```python
from build123d import *

# Parameters (mm, degrees)
SKETCH1_W = 9.525
SKETCH1_H = 3.175


with BuildPart() as part:
    # Sketch1 → Revolve2 (revolve)
    with BuildSketch(Plane.XY, mode=Mode.PRIVATE) as revolve2_sk:
        Polygon((0, 9.525), (0, 0), (31.75, 0), (31.75, 7.62), (31.75, 9.525), align=None)
        Polygon((31.75, 7.62), (31.75, 0), (38.1, 0), (38.1, 6.35), (38.1, 7.62), align=None)
        Polygon((38.1, 6.35), (38.1, 0), (47.625, 0), (47.625, 5.715), (47.625, 6.35), align=None)
        Polygon((47.625, 5.715), (47.625, 0), (57.15, 0), (57.15, 4.445), (57.15, 5.715), align=None)
        Polygon((57.15, 4.445), (57.15, 0), (66.675, 0), (66.675, 3.175), (66.675, 4.445), align=None)
        with Locations((71.4375, 1.5875)):
            Rectangle(SKETCH1_W, SKETCH1_H)
    revolve(revolve2_sk.sketch.rotate(Axis((0, 0, 0), (1, 0, 0)), 90), axis=Axis((0, 0, 0), (1, 0, 0)))


solid = part.part
```
Source: CAD feature listing. Evaluate the final solid. Frame: model axes, mm. A direction names the side the tool comes from. Round coordinates to 2 decimals unless told otherwise and drop trailing zeros. Loops run counter-clockwise (first coordinate to the right, second up) from the corner with the lowest first, then second, coordinate; pieces in that order, holes last. Notation, with made-up numbers: M 73.5,23 L 90.5,23 A25 ccw 90.5,51 Z; hole C 58,42 d7. An arc over 180 degrees is marked long. Use a Markdown table: item, result. Add a question column.
1. Cut plane C-C, the plane x = 43. Output: boundary loops of the cut face in (y, z).
2. Cut plane A-A, the plane z = 0. Output: boundary loops of the cut face in (x, y) (3 decimals), and give its area (3 significant figures).
3. Set-up query: faces 1 (the cylindrical face through (71.5, 1.93, -2.52)), 2 (the flat face through (76.2, 0, 0)). Return all of +Z, -Z, +X, -X, +Y, -Y with unobstructed straight access to the full face (end or side cutting, diameter ignored); none if empty.
4. Contact query for flat-ended pins moving along their axis: pin 1 (1 mm diameter, centred on y = -0.5, z = 4, fed in from +X) (3 decimals); pin 2 (6 mm diameter, centred on x = 67.5, z = -4, fed in from +Y); pin 3 (4 mm diameter, centred on y = 0.5, z = 7, fed in from +X). Output: stop coordinate, or through.
5. Cut plane D-D, the plane x = 34. Output: boundary loops of the cut face in (y, z).
6. Ray query, line 1 along X through (y, z) = (3.5, 3.25); line 2 along X through (y, z) = (-5, -4); line 3 along Z through (x, y) = (23, -0.25). Return the intervals inside material, ascending. Write a range as [from, to].
Solution:
| question | item | result |
|---|---|---|
| 1 | outline | C 0,0 d12.7 |
| 2 | outline | M 0,-9.525 L 31.75,-9.525 L 31.75,-7.62 L 38.1,-7.62 L 38.1,-6.35 L 47.625,-6.35 L 47.625,-5.715 L 57.15,-5.715 L 57.15,-4.445 L 66.675,-4.445 L 66.675,-3.175 L 76.2,-3.175 L 76.2,3.175 L 66.675,3.175 L 66.675,4.445 L 57.15,4.445 L 57.15,5.715 L 47.625,5.715 L 47.625,6.35 L 38.1,6.35 L 38.1,7.62 L 31.75,7.62 L 31.75,9.525 L 0,9.525 Z |
| 2 | area | 1,080 mm2 |
| 3 | face 1 | +X |
| 3 | face 2 | +Z, -Z, +X, +Y, -Y |
| 4 | pin 1 | stops at x = 66.675 |
| 4 | pin 2 | stops at y = 4.3 |
| 4 | pin 3 | stops at x = 57.15 |
| 5 | outline | C 0,0 d15.24 |
| 6 | line 1 | x = [0, 57.15] |
| 6 | line 2 | x = [0, 38.1] |
| 6 | line 3 | z = [-9.52, 9.52] |
